Verification items for this drawing (mm, ordinates from the low corner). Coordinates: 2 decimals unless noted, no trailing zeros. Order: outer loops, then holes, each group sorted by start corner. A loop starts at its lowest first (then second) coordinate and runs counter-clockwise, first axis right, second up. Notation, with made-up numbers: M 45,-14 L 74,-14 A13 cw 74,10 Z; hole C -39.5,-13 d1. An arc over 180 degrees is marked long. Write item = value, one per line.
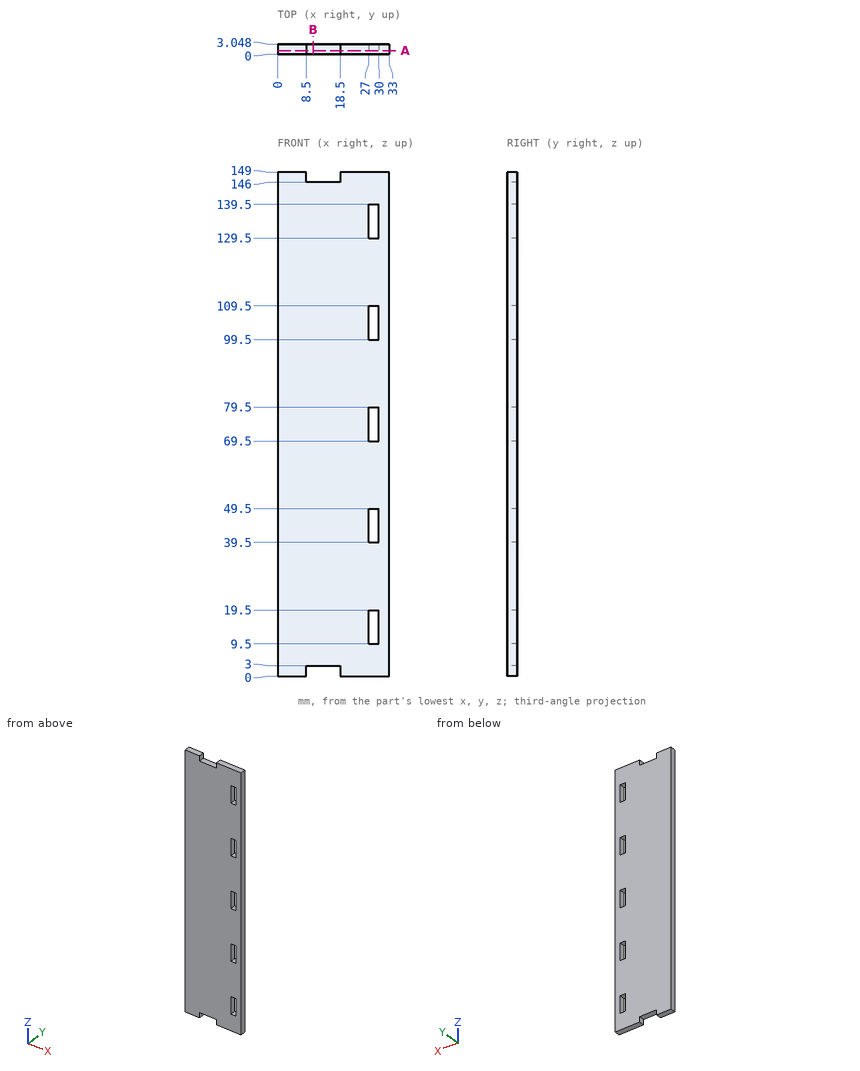
Item 1: Sectioned sample at B-B, the plane x = 10.5. Enter the section's corners in (y, z), then the cut area to 3 significant figures.
Report:
outline = M 0,3 L 3.05,3 L 3.05,146 L 0,146 Z
area = 436 mm^2
Item 2: Scan lines: L1, parallel to Z at x = 28.5, y = 0.7; L2, parallel to X at y = 0.4, z = 138; L3, parallel to Z at x = 13, y = 1.7. Record each from-to range of solid material in increasing order. Write a range as from..to.
Report:
L1 = 0..9.5, 19.5..39.5, 49.5..69.5, 79.5..99.5, 109.5..129.5, 139.5..149
L2 = 0..27, 30..33
L3 = 3..146
Item 3: Gauge pin test, flat end, axial feed: pin 1 (1 mm diameter, centred on x = 13.5, y = 2.5, fed in from -Z). Record the tip position at first contact, or that the pin passes through.
Report:
pin_1 = 3
Item 4: Sectioned sample at A-A, the plane y = 1.1. Give the number of separate pieces and of enclosed holes in the cut face, then the cut area to 3 significant figures.
Report:
separate_pieces = 1
enclosed_holes = 5
area = 4,710 mm^2
